from build123d import *

# Parameters (mm, degrees)
SKETCH1_R                = 1.25
BOSS_EXTRUDE1_DEPTH      = 11
BOSS_EXTRUDE2_DEPTH      = 2
BOSS_EXTRUDE2_DEPTH_BACK = 8
SKETCH1_2_R              = 1.25


with BuildPart() as part:
    # Sketch1 → Boss-Extrude1 (new body)
    with BuildSketch(Plane(origin=(0, 0, 0), x_dir=(1, 0, 0), z_dir=(0, 1, 0))):
        Polygon((-2.886751346, 0), (-1.443375673, -2.5), (1.443375673, -2.5), (2.886751346, 0), (1.443375673, 2.5), (-1.443375673, 2.5), align=None)
        with Locations(Location((0, 0, 0), (0, 0, 270))):
            Circle(SKETCH1_R, mode=Mode.SUBTRACT)
    extrude(amount=BOSS_EXTRUDE1_DEPTH)

    # Sketch1_2 → Boss-Extrude2 (add, two sides: drawn at the far end of the back side and taken through both)
    with BuildSketch(Plane(origin=(0, 0, 0), x_dir=(1, 0, 0), z_dir=(0, 1, 0)).offset(-BOSS_EXTRUDE2_DEPTH_BACK)):
        with Locations(Location((0, 0, 0), (0, 0, 270))):
            Circle(SKETCH1_2_R)
    extrude(amount=BOSS_EXTRUDE2_DEPTH + BOSS_EXTRUDE2_DEPTH_BACK)


solid = part.part
Geometry: final body of the model. Coordinates: model frame, mm. A direction names the side the tool comes from. Round coordinates to 2 decimals unless told otherwise and drop trailing zeros. Loops run counter-clockwise (first coordinate to the right, second up) from the corner with the lowest first, then second, coordinate; pieces in that order, holes last. Notation, with made-up numbers: M 32,39 L 69,39 A30 cw 69,69 Z; hole C 66.25,-18.5 d9. An arc over 180 degrees is marked long. One line per question, with ' | ' between items.
(1) Access query for faces 1 (the cylindrical face through (-1.22, 6.44, -0.27)), 2 (the flat face through (2.155, 5.423, 1.267)), 3 (the cylindrical face through (-1.22, -4.06, -0.27)). Directions: +Z, -Z, +X, -X, +Y, -Y. A direction counts if a zero-diameter tool reaches every point of the face in a straight line with its end or side. Return the directions, or none.
Check result:
face 1: +Y | face 2: +Z, +X, +Y, -Y | face 3: -Y
(2) Material intervals for line 1 along Y through (x, z) = (0.3, 1.4); line 2 along Y through (x, z) = (0, 0.5); line 3 along X through (y, z) = (2.25, -0.3), sorted ascending. Write a range as from..to.
Check result:
line 1: y = 0..11 | line 2: y = -8..2 | line 3: x = -2.71..-1.21, 1.21..2.71
(3) Contact query for flat-ended pins moving along their axis: P1, Ø3, axis at x = -2, y = -2, coming from the +Z side; P2, Ø1.5, axis at x = 1, y = -5.5, coming from the +Z side; P3, Ø1.2, axis at x = -0.5, z = 0, coming from the +Y side. Output: stop coordinate, or through.
Check result:
P1: stops at z = 1.15 | P2: stops at z = 1.22 | P3: stops at y = 2
(4) Cut plane A-A on y = 8. Return the cut outline in (x, z).
Check result:
outline: M -2.89,0 L -1.44,-2.5 L 1.44,-2.5 L 2.89,0 L 1.44,2.5 L -1.44,2.5 Z; hole C 0,0 d2.5
(5) Cut plane B-B on x = 0. Return the cut outline in (y, z), plus the area to 3 significant figures.
Check result:
outline: M -8,-1.25 L 0,-1.25 L 0,-2.5 L 11,-2.5 L 11,-1.25 L 2,-1.25 L 2,1.25 L 11,1.25 L 11,2.5 L 0,2.5 L 0,1.25 L -8,1.25 Z | area: 52.5 mm2
(6) Cut plane C-C on z = 0.95. Return the cut outline in (x, y), plus the area to 3 significant figures.
Check result:
outline: M -2.34,0 L -0.81,0 L -0.81,-8 L 0.81,-8 L 0.81,0 L 2.34,0 L 2.34,11 L 0.81,11 L 0.81,2 L -0.81,2 L -0.81,11 L -2.34,11 Z | area: 49.8 mm2
